CAD build for the part. Positions are in the model's coordinates, mm. Face numbers are marked on the shaded views. A direction names the side the tool comes from. Round coordinates to 2 decimals unless told otherwise and drop trailing zeros. Order: outer loops, then holes, each group sorted by start corner. A loop starts at its lowest first (then second) coordinate and runs counter-clockwise, first axis right, second up.
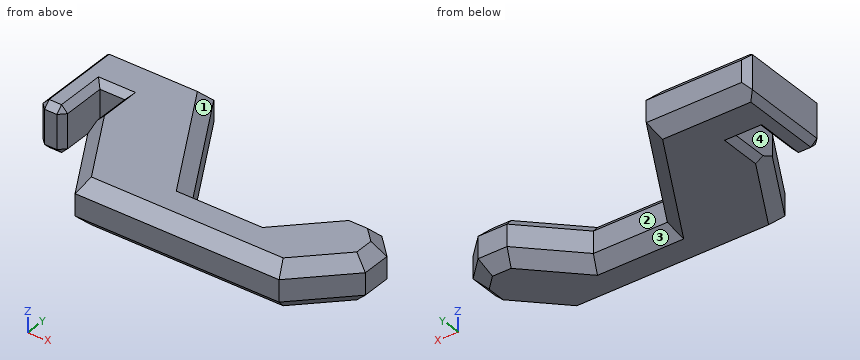
```python
from build123d import *

# Parameters (mm, degrees)
F1_DEPTH = 5.969
F2_W     = 3.175
F2_H     = 6.35
F3_DEPTH = 5.97
F4_SIZE  = 0.79375
F5_SIZE  = 1.58749


# Not quite as in the source:
# - a fillet or chamfer is up to 0.001 mm smaller than in the source, because OpenCascade refuses the exact size


with BuildPart() as f1:
    # F0 (on Top) → F1 (new body)
    with BuildSketch(Plane.XY):
        Polygon((13.0595644766, 0), (0, 0), (0, -12.7), (6.35, -12.7), (11.849261314, -22.225), (38.1, -22.225), (44.45, -15.875), (44.45, -12.1552561211), (41.8197438789, -9.525), (38.1, -9.525), (31.75, -15.875), (22.225, -15.875), align=None)
    extrude(amount=F1_DEPTH)

    # F2 (on face) → F3 (cut, through all)
    with BuildSketch(Plane.XY.offset(5.969)):
        with Locations((4.7625, -9.525)):
            Rectangle(F2_W, F2_H)
    extrude(amount=-F3_DEPTH, mode=Mode.SUBTRACT)

    # F4
    f4_edges = [f1.edges().sort_by_distance(p)[0] for p in [
        (0, 0, 2.9845),
        (0, -12.7, 2.9845),
        (0, -6.35, 0),
        (0, -6.35, 5.969),
        (1.5875, -12.7, 0),
        (3.175, -12.7, 2.9845),
        (1.5875, -12.7, 5.969),
        (3.175, -9.525, 5.969),
        (3.175, -9.525, 0),
        (4.7625, -6.35, 5.969),
        (6.35, -9.525, 5.969),
        (4.7625, -6.35, 0),
        (6.35, -9.525, 0),
    ]]
    chamfer(f4_edges, length=F4_SIZE)

    # F5 (size 1.5875 in the source; OpenCascade refuses exactly that, so slightly less here)
    f5_edges = [f1.edges().sort_by_distance(p)[0] for p in [
        (6.926657, 0, 0),
        (17.642282, -7.9375, 0),
        (26.9875, -15.875, 0),
        (34.925, -12.7, 0),
        (39.959872, -9.525, 0),
        (43.134872, -10.840128, 0),
        (44.45, -14.015128, 0),
        (41.275, -19.05, 0),
        (24.974631, -22.225, 0),
        (9.496506, -18.149908, 0),
        (9.496506, -18.149908, 5.969),
        (24.974631, -22.225, 5.969),
        (41.275, -19.05, 5.969),
        (44.45, -14.015128, 5.969),
        (43.134872, -10.840128, 5.969),
        (34.925, -12.7, 5.969),
        (39.959872, -9.525, 5.969),
        (26.9875, -15.875, 5.969),
        (17.642282, -7.9375, 5.969),
        (6.926657, 0, 5.969),
    ]]
    chamfer(f5_edges, length=F5_SIZE)


solid = f1.part
```
1. Cut at D-D, the plane x = 15. Write the cut outline in (y, z) (1 decimal), and give its area (3 significant figures).
2. Drill centre lines: line 1 (X direction, y = -10.75, z = 3.7) (3 decimals); line 2 (X direction, y = -8.5, z = 2.75) (3 decimals); line 3 (X direction, y = -14, z = 5.6). Where is each one in solid material? Low to high.
3. Tool access for the marked faces 1, 2, 3 and 4: list every direction of +Z, -Z, +X, -X, +Y, -Y with a clear straight run to the whole face (end or side of a thin tool).
4. Cut at B-B, the plane z = 3.5. Write the cut outline in (x, y) (3 decimals), and give its area (3 significant figures).
5. Cut at C-C, the plane y = -3.75. Write the cut outline in (x, z).
6. Pin check, flat tips, straight feed: P1, Ø3, axis at x = 28.5, z = 3.5, coming from the +Y side (3 decimals); P2, Ø1.4, axis at x = 39.5, z = 3.5, coming from the +Y side (3 decimals); P3, Ø1.5, axis at y = -7, z = 2.5, coming from the +X side. Stop position of each tip, or through.
Outcome:
1. outline: (-22.2, 1.6) - (-20.6, 0) - (-6.5, 0) - (-3.4, 1.6) - (-3.4, 4.4) - (-6.5, 6) - (-20.6, 6) - (-22.2, 4.4) - close
1. area: 105 mm2
2. line 1: x = 0 to 3.175, 6.35 to 19.266, 36.875 to 43.045
2. line 2: x = 0 to 3.175, 6.35 to 17.967
2. line 3: x = 8.51 to 19.74, 35.35 to 43.23
3. face 1: +Z, +Y
3. face 2: +Z, -Z, +Y
3. face 3: -Z, +Y
3. face 4: +Z, -Z, -Y
4. outline: (0, -11.906) - (0.794, -12.7) - (2.381, -12.7) - (3.175, -11.906) - (3.175, -6.35) - (6.35, -6.35) - (6.35, -12.7) - (11.849, -22.225) - (38.1, -22.225) - (44.45, -15.875) - (44.45, -12.155) - (41.82, -9.525) - (38.1, -9.525) - (31.75, -15.875) - (22.225, -15.875) - (13.06, 0) - (0.794, 0) - (0, -0.794) - close
4. area: 491 mm2
5. outline: (0, 0.79) - (0.79, 0) - (13.39, 0) - (15.22, 1.59) - (15.22, 4.38) - (13.39, 5.97) - (0.79, 5.97) - (0, 5.18) - close
6. P1: stops at y = -15.875
6. P2: stops at y = -9.525
6. P3: stops at x = 17.53
